from build123d import *

# Parameters (mm, degrees)
SKETCH2_R                       = 127
EXTRUDE1_DEPTH                  = 12.7
F_11_16_0_6875_DIAMETER_HOLE1_D = 17.4625
CIRPATTERN1_COUNT               = 8


with BuildPart() as part:
    # Sketch2 → Extrude1 (new body)
    with BuildSketch(Plane(origin=(0, 0, 0), x_dir=(1, 0, 0), z_dir=(0, 1, 0))):
        Circle(SKETCH2_R)
    extrude(amount=EXTRUDE1_DEPTH)

    # 11_16 _0.6875_ Diameter Hole1 (through all)
    with Locations(Plane(origin=(0, 12.7, 0), x_dir=(-1, 0, 0), z_dir=(0, 1, 0))):
        with Locations((-101.6, 0)):
            f_11_16_0_6875_diameter_hole1 = Hole(F_11_16_0_6875_DIAMETER_HOLE1_D / 2)

    # CirPattern1: 11_16 _0.6875_ Diameter Hole1 ×8 about axis
    cirpattern1_axis = Axis((0, 0, 0), (0, 1, 0))
    for i in range(1, CIRPATTERN1_COUNT):
        add(f_11_16_0_6875_diameter_hole1.rotate(cirpattern1_axis, i * 360 / CIRPATTERN1_COUNT), mode=Mode.SUBTRACT)


solid = part.part
Can you work these out from the model? Positions are in its coordinate system, mm. Give positions to 0.01 mm unless a question says otherwise; leave off trailing zeros. Write each loop counter-clockwise with the first axis right and the second up, starting at its lowest first coordinate (ties: lowest second). Pieces come first, ordered by that corner, then holes. Notation, with made-up numbers: M -11.75,45.25 L 2.25,45.25 A24 ccw 2.25,69.25 Z; hole C -16.75,57 d10. An arc over 180 degrees is marked long. Answer in a Markdown table with one row per item. Add a question column.
Item 1: Imagine slicing it at B-B, the plane x = 0. Write out the boundary of the cut face in (y, z).
Item 2: Please list where these lines run through material, in increasing order: L1, parallel to X at y = 9.75, z = -77.5; L2, parallel to Z at x = 3.5, y = 11; L3, parallel to X at y = 12, z = 66.
Item 3: Imagine slicing it at A-A, the plane z = -101.6. Write out the boundary of the cut face in (x, y).
Item 4: Imagine slicing it at C-C, the plane z = 0. Write out the boundary of the cut face in (x, y), plus the area to 3 significant figures.
Item 5: We'd pull the mould along Z, two halves only. Please class faces 1 (the cylindrical face through (-0.384, 6.261, 92.877)), 2 (the flat face through (-2, 0, -2)), 3 (the cylindrical face through (-27.53, 6.26, 123.98)): released by +Z, released by -Z, zero draft, split by the parting line, or undercut.
Item 6: For pin 1 Ø14 at (x, z) = (101.6, 0) entering from +Y; pin 2 Ø22.5 at (x, z) = (71.84, -71.84) entering from +Y; pin 3 Ø2 at (y, z) = (11, 87.5) entering from +X; pin 4 Ø4 at (x, y) = (-37, 8.5) entering from +Z, each with a flat end and sliding along its axis, tell me the tip position at first contact or that it passes through.
Item 7: Imagine slicing it at D-D, the plane x = -101.6. Write out the boundary of the cut face in (y, z), plus the area to 3 significant figures.
Evaluation:
| question | item | result |
|---|---|---|
| 1 | outline | M 0,-127 L 12.7,-127 L 12.7,-110.33 L 0,-110.33 Z; M 0,-92.87 L 12.7,-92.87 L 12.7,92.87 L 0,92.87 Z; M 0,110.33 L 12.7,110.33 L 12.7,127 L 0,127 Z |
| 2 | L1 | x = -100.61 to -78.49, -65.19 to 65.19, 78.49 to 100.61 |
| 2 | L2 | z = -126.95 to -109.6, -93.6 to 93.6, 109.6 to 126.95 |
| 2 | L3 | x = -108.5 to -78.33, -65.35 to 65.35, 78.33 to 108.5 |
| 3 | outline | M -76.2,0 L -8.73,0 L -8.73,12.7 L -76.2,12.7 Z; M 8.73,0 L 76.2,0 L 76.2,12.7 L 8.73,12.7 Z |
| 4 | outline | M -127,0 L -110.33,0 L -110.33,12.7 L -127,12.7 Z; M -92.87,0 L 92.87,0 L 92.87,12.7 L -92.87,12.7 Z; M 110.33,0 L 127,0 L 127,12.7 L 110.33,12.7 Z |
| 4 | area | 2,780 mm² |
| 5 | face 1 | undercut |
| 5 | face 2 | zero draft |
| 5 | face 3 | split by the parting line |
| 6 | pin 1 | passes through |
| 6 | pin 2 | stops at y = 12.7 |
| 6 | pin 3 | stops at x = 92.99 |
| 6 | pin 4 | stops at z = 122.08 |
| 7 | outline | M 0,-76.2 L 12.7,-76.2 L 12.7,-8.73 L 0,-8.73 Z; M 0,8.73 L 12.7,8.73 L 12.7,76.2 L 0,76.2 Z |
| 7 | area | 1,710 mm² |
